Read the model definition and answer for the solid it produces. Units are mm, in the model's axes. Round coordinates to 2 decimals unless told otherwise and drop trailing zeros. Write each loop counter-clockwise with the first axis right and the second up, starting at its lowest first coordinate (ties: lowest second). Pieces come first, ordered by that corner, then holes. Notation, with made-up numbers: (4, 14.5) - (22, 14.5) arc R25 cw to (22, 48.5) - close; hole circle Ø3 at (83.5, 17). An arc over 180 degrees is marked (long way). Answer as CSV lines item,"result". Start each with the question number.
1) Find section A-A on z = 672.5. Determine the outline of the cut face in (x, y).
2) Consider line 1 along X through (y, z) = (-4.75, 732); line 2 along Y through (x, z) = (1, 377); line 3 along X through (y, z) = (-0.5, 567.5). Determine where each line is inside the solid, lowest interval first.
3) Each of these flat-tipped pins is pushed along its axis until it touches: pin 1 (1 mm diameter, centred on x = 4, z = 561.5, fed in from -Y); pin 2 (4 mm diameter, centred on x = -3.5, z = 315, fed in from -Y); pin 3 (4 mm diameter, centred on x = 4, y = 1.5, fed in from +Z); pin 4 (2 mm diameter, centred on y = 3.5, z = 188, fed in from +X). Where does it stop, or does it pass through?
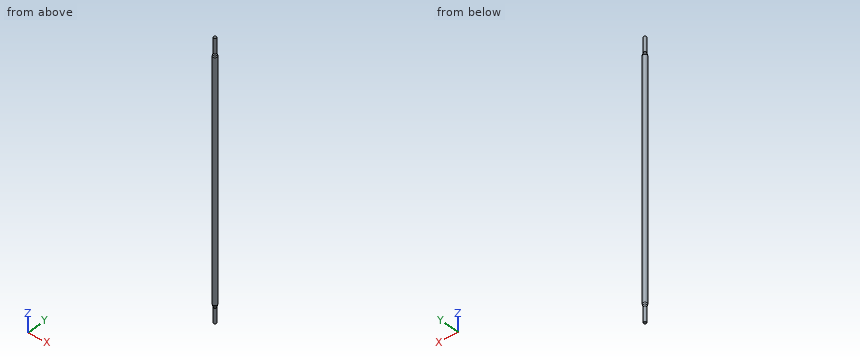
from build123d import *

# Parameters (mm, degrees)
SKETCH1_R           = 4
BOSS_EXTRUDE1_DEPTH = 50
SKETCH2_R           = 6.25
BOSS_EXTRUDE2_DEPTH = 700
SKETCH3_R           = 4
BOSS_EXTRUDE3_DEPTH = 50
FILLET1_R           = 10
FILLET2_R           = 10


with BuildPart() as part:
    # Sketch1 → Boss-Extrude1 (new body)
    with BuildSketch(Plane.XY):
        Circle(SKETCH1_R)
    extrude(amount=BOSS_EXTRUDE1_DEPTH)

    # Sketch2 → Boss-Extrude2 (add)
    with BuildSketch(Plane.XY.offset(50)):
        Circle(SKETCH2_R)
    extrude(amount=BOSS_EXTRUDE2_DEPTH)

    # Sketch3 → Boss-Extrude3 (add)
    with BuildSketch(Plane.XY.offset(750)):
        Circle(SKETCH3_R)
    extrude(amount=BOSS_EXTRUDE3_DEPTH)

    # Fillet1
    # the kernel refuses this fillet: 10 mm, written as the material it adds along each edge
    with BuildSketch(Plane(origin=(0, 0, 750), x_dir=(1, 0, 0), z_dir=(0, -1, 0))) as fillet1_piece_1:
        with BuildLine():
            CenterArc((14, 6.31961233), FILLET1_R, 180, 39.194967426)
            Line((4, 6.31961233), (3.8, 6.31961233))
            Line((3.8, 6.31961233), (3.8, 0))
            Line((3.8, 0), (4, -0.2))
            ThreePointArc((4, -0.2), (5.125, -0.2), (6.095, -0.126392247))
            Line((6.095, -0.126392247), (6.25, 0))
        make_face()
    revolve(axis=Axis((0, 0, 750), (0, 0, 1)))
    with BuildSketch(Plane(origin=(0, 0, 50), x_dir=(1, 0, 0), z_dir=(0, -1, 0))) as fillet1_piece_2:
        with BuildLine():
            CenterArc((14, -6.31961233), FILLET1_R, 140.805032574, 39.194967426)
            Line((4, -6.31961233), (3.8, -6.31961233))
            Line((3.8, -6.31961233), (3.8, 0))
            Line((3.8, 0), (4, 0.2))
            ThreePointArc((4, 0.2), (5.125, 0.2), (6.095, 0.126392247))
            Line((6.095, 0.126392247), (6.25, 0))
        make_face()
    revolve(axis=Axis((0, 0, 50), (0, 0, 1)))

    # Fillet2
    fillet2_edges = [part.edges().sort_by_distance(p)[0] for p in [
        (-6.25, 0, 50),
        (-6.25, 0, 750),
    ]]
    fillet(fillet2_edges, radius=FILLET2_R)


solid = part.part
Check values:
1,outline,"circle Ø12.5 at (0, 0)"
2,line 1,"x = -4.06 to 4.06"
2,line 2,"y = -6.17 to 6.17"
2,line 3,"x = -6.23 to 6.23"
3,pin 1,"stops at y = -5.18"
3,pin 2,"stops at y = -6.07"
3,pin 3,"stops at z = 800"
3,pin 4,"stops at x = 5.73"
